```python
from build123d import *

# Parameters (mm, degrees)
F1_DEPTH    = 0.762
F3_DEPTH    = 8.763
F4_R        = 6.2484
F5_R        = 2.0955
F6_DEPTH    = 0.763
F7_T        = 0.762
F7_T3_DEPTH = 18.68884375
F7_T5_DEPTH = 2.286
F7_T8_ANGLE = 180.000000001
F8_DEPTH    = 0.763
F9_R        = 0.762


# Not quite as in the source:
# - a shell that OpenCascade refuses in one call is made with other operations: the cavity is built on its own and cut out


with BuildPart() as f1:
    # F0 (on Front) → F1 (new body)
    with BuildSketch(Plane.XZ):
        with BuildLine():
            ThreePointArc((12.7, 12.7), (6.35, 19.05), (0, 12.7))
            Line((0, 12.7), (0, -12.7))
            ThreePointArc((0, -12.7), (6.35, -19.05), (12.7, -12.7))
            Line((12.7, -12.7), (12.7, -7.9375))
            Line((12.7, -7.9375), (17.4625, -7.9375))
            ThreePointArc((17.4625, -7.9375), (25.4, 0), (17.4625, 7.9375))
            Line((17.4625, 7.9375), (12.7, 7.9375))
            Line((12.7, 7.9375), (12.7, 12.7))
        make_face()
    extrude(amount=-F1_DEPTH)

    # F2 (on face) → F3 (join)
    with BuildSketch(Plane.XZ):
        with BuildLine():
            Line((17.16484375, 6.25078125), (0, 6.25078125))
            Line((0, 6.25078125), (0, -6.25078125))
            Line((0, -6.25078125), (17.16484375, -6.25078125))
            ThreePointArc((17.16484375, -6.25078125), (23.415625, 0), (17.16484375, 6.25078125))
        make_face()
    extrude(amount=F3_DEPTH)

    # F4
    f4_edges = [f1.edges().sort_by_distance(p)[0] for p in [
        (8.582422, -8.763, 6.250781),
    ]]
    fillet(f4_edges, radius=F4_R)

    # F5 (on face) → F6 (cut, through all)
    with BuildSketch(Plane.XZ):
        with Locations((6.35, 12.7)):
            Circle(F5_R)
        with Locations((6.35, -12.7)):
            Circle(F5_R)
    extrude(amount=-F6_DEPTH, mode=Mode.SUBTRACT)

    # F7: shell of thickness 0.762, made by hand


with BuildPart() as f7_core1:
    # F7_t2: copy of F1
    add(f1.part)

    # the walls: a layer under each face that stays
    f7_faces = [f7_core1.faces().sort_by_distance(p)[0] for p in [
        (8.582421875, -1.2573, -6.25078125),
        (8.582421875, -6.9328860116, -4.4206672616),
        (4.2333333333, 0, -12.7),
        (8.5836125, -8.763, 0),
        (6.35, 0.381, -19.05),
        (8.582421875, -6.9328860116, 4.4206672616),
        (12.7, 0.762, 0),
        (8.582421875, -1.2573, 6.25078125),
        (6.35, 0.381, 19.05),
        (23.415625, -1.2573, 0),
        (21.5855110116, -6.9328860116, 0),
        (12.7, 0.381, -10.31875),
        (15.08125, 0.381, -7.9375),
        (25.4, 0.381, 0),
        (15.08125, 0.381, 7.9375),
        (12.7, 0.381, 10.31875),
        (4.2545, 0.381, -12.7),
        (4.2545, 0.381, 12.7),
    ]]
    thicken(f7_faces, amount=-F7_T, mode=Mode.SUBTRACT)

    # F7_s4 → F7_t3 (cut)
    with BuildSketch(Plane.YZ.offset(-0.762)):
        Polygon((-0.00762, -6.25840125), (0, -5.48878125), (0.762, -5.48878125), (0.762, -6.25078125), align=None)
        Polygon((-0.00762, 6.25840125), (0.762, 6.25078125), (0.762, 5.48878125), (0, 5.48878125), align=None)
    extrude(amount=F7_T3_DEPTH, mode=Mode.SUBTRACT)

    # F7_s6 → F7_t5 (cut)
    with BuildSketch(Plane.XZ.offset(-1.524)):
        Polygon((12.70762, -7.94512), (11.938, -7.9375), (11.938, -7.1755), (12.7, -7.1755), align=None)
        Polygon((12.70762, 7.94512), (12.7, 7.1755), (11.938, 7.1755), (11.938, 7.9375), align=None)
    extrude(amount=F7_T5_DEPTH, mode=Mode.SUBTRACT)

    # F7_s7 → F7_t8 (revolve, cut)
    with BuildSketch(Plane.YZ.offset(17.16484375)):
        Polygon((-0.00762, -6.25840125), (0.762, -6.25078125), (0.762, -5.48878125), (0, -5.48878125), align=None)
    revolve(axis=Axis((17.16484375, 0, 0), (0, -1, 0)), revolution_arc=F7_T8_ANGLE, mode=Mode.SUBTRACT)


with BuildPart() as f1_1:
    add(f1.part)

    # what is left inside the walls is the cavity
    f7_cavity = [f7_core1.part.solids().sort_by_distance(p)[0] for p in [
        (11.326812, -0.00762, -1.829594),
    ]]
    add(f7_cavity, mode=Mode.SUBTRACT)

    # F8 (cut, through all): a face of the model
    f8_faces = [f1_1.faces().sort_by_distance(p)[0] for p in [
        (10.7728031168, 0, 0),
    ]]
    extrude(f8_faces, amount=-F8_DEPTH, mode=Mode.SUBTRACT)

    # F9
    f9_edges = [f1_1.edges().sort_by_distance(p)[0] for p in [
        (8.582422, 0, 6.250781),
        (8.582422, 0.762, 5.488781),
    ]]
    fillet(f9_edges, radius=F9_R)


solid = f1_1.part
```
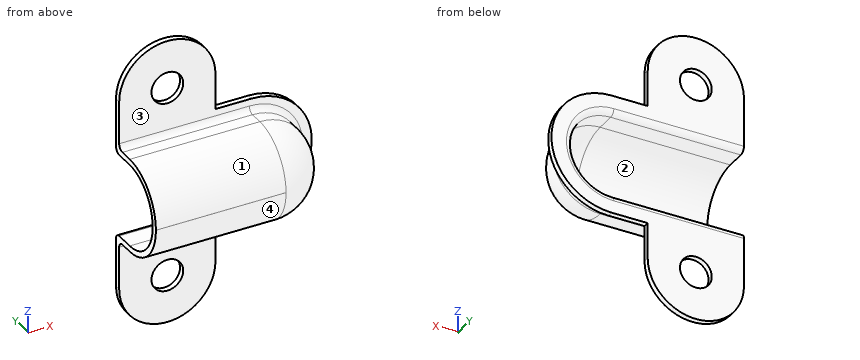
Model file for the job. Use its own axes, mm. Face numbers are marked on the shaded views. Round coordinates to 2 decimals unless told otherwise and drop trailing zeros. Use one line per item in the form item = value.
Item 1: Cut at A-A, the plane x = 6.35. Give the number of separate pieces and of enclosed holes in the cut face, and give its area (3 significant figures).
Returned:
separate_pieces = 3
enclosed_holes = 0
area = 32.2 mm^2
Item 2: Pull direction Z, two halves, no side cores. Call the marked faces 1, 2, 3 and 4: released by +Z, released by -Z, zero draft, split by the parting line, or undercut.
Returned:
face_1 = released by +Z
face_2 = undercut
face_3 = zero draft
face_4 = released by -Z
Item 3: Flat gauge pins, fed straight in: pin 1 Ø1 at (x, z) = (9.5, 14) entering from -Y; pin 2 Ø4 at (x, z) = (16.5, -0.5) entering from -Y; pin 3 Ø0.9 at (x, y) = (6.5, -2) entering from -Z; pin 4 Ø12 at (x, z) = (23, -11) entering from -Y. Where does each tip first touch, or does it go through?
Returned:
pin_1 = 0
pin_2 = -8.76
pin_3 = -6.25
pin_4 = -0.25
Item 4: Drill centre lines: line 1 (Z direction, x = 6.35, y = 0.25); line 2 (Z direction, x = 6.35, y = 0.4); line 3 (Z direction, x = 6.5, y = -1.5). Where is each one in solid material? Low to high.
Returned:
line_1 = -19.05 to -14.8, -10.6 to -5.53, 5.53 to 10.6, 14.8 to 19.05
line_2 = -19.05 to -14.8, -10.6 to -5.6, 5.6 to 10.6, 14.8 to 19.05
line_3 = -6.25 to -5.49, 5.49 to 6.25
